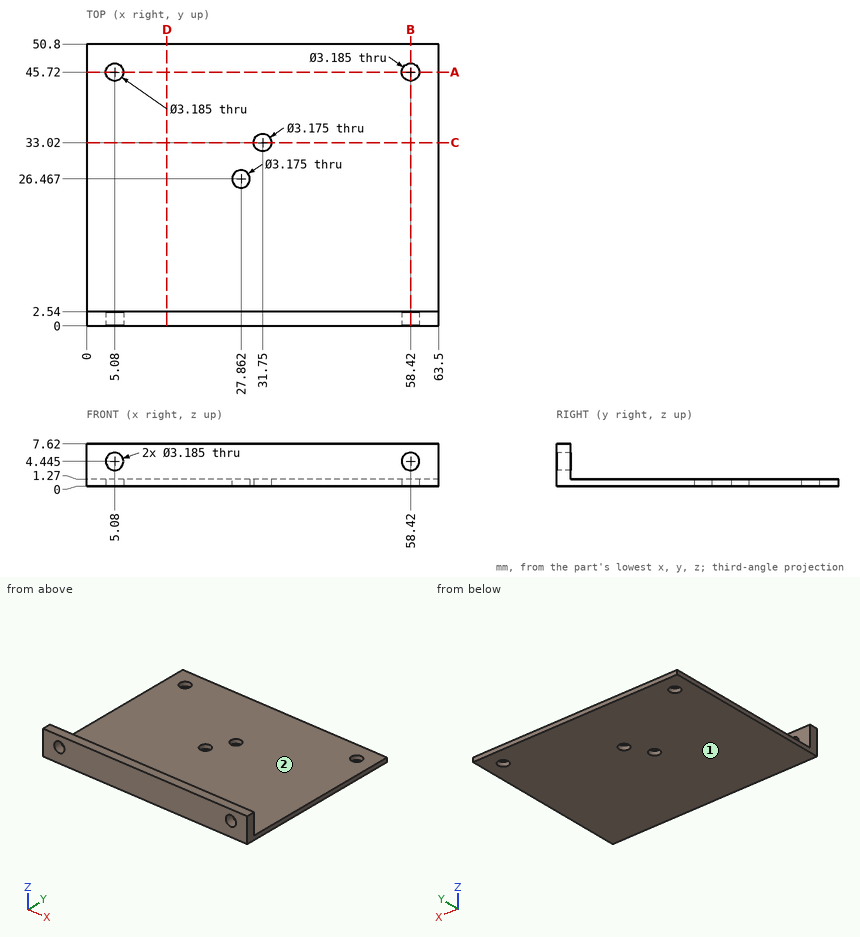
Job drawing, mm, ordinate dimensions from the low corner. One solid piece. A direction names the side the tool comes from. Coordinates: 2 decimals unless noted, no trailing zeros. Write each loop counter-clockwise with the first axis right and the second up, starting at its lowest first coordinate (ties: lowest second). Pieces come first, ordered by that corner, then holes.
Item 1: Slice it at B-B (x = 58.42). Write the cut outline in (y, z).
Item 2: Pin check, flat tip, straight feed: pin 1 (4 mm diameter, centred on x = 31.75, y = 33.02, fed in from +Z). Stop position of the tip, or through.
Item 3: Slice it at A-A (y = 45.72). Write the cut outline in (x, z).
Item 4: Slice it at D-D (x = 14.5). Write the cut outline in (y, z).
Item 5: Probe line 1 (X direction, y = 45.72, z = 0.5); line 2 (Y direction, x = 31.75, z = 0.75); line 3 (Z direction, x = 5.08, y = 0.6). List the from-to ranges inside material, lowest first.
Item 6: Which spindle directions (+Z, -Z, +X, -X, +Y, -Y) get a long thin tool onto all of the face, cutting with end or side? Do the marked faces 1 and 2. Say none if no direction does.
Item 7: Slice it at C-C (y = 33.02). Write the cut outline in (x, z).
Results found:
1. outline: (0, 0) - (44.13, 0) - (44.13, 1.27) - (2.54, 1.27) - (2.54, 2.85) - (0, 2.85) - close; (0, 6.04) - (2.54, 6.04) - (2.54, 7.62) - (0, 7.62) - close; (47.31, 0) - (50.8, 0) - (50.8, 1.27) - (47.31, 1.27) - close
2. pin 1: stops at z = 1.27
3. outline: (0, 0) - (3.49, 0) - (3.49, 1.27) - (0, 1.27) - close; (6.67, 0) - (56.83, 0) - (56.83, 1.27) - (6.67, 1.27) - close; (60.01, 0) - (63.5, 0) - (63.5, 1.27) - (60.01, 1.27) - close
4. outline: (0, 0) - (50.8, 0) - (50.8, 1.27) - (2.54, 1.27) - (2.54, 7.62) - (0, 7.62) - close
5. line 1: x = 0 to 3.49, 6.67 to 56.83, 60.01 to 63.5
5. line 2: y = 0 to 31.43, 34.61 to 50.8
5. line 3: z = 0 to 2.85, 6.04 to 7.62
6. face 1: -Z, +X, -X, +Y, -Y
6. face 2: +Z, +X, -X, +Y
7. outline: (0, 0) - (30.16, 0) - (30.16, 1.27) - (0, 1.27) - close; (33.34, 0) - (63.5, 0) - (63.5, 1.27) - (33.34, 1.27) - close
